from build123d import *

# Parameters (mm, degrees)
SKETCH_1_W          = 25
SKETCH_1_H          = 10
EXTRUDE_1_DEPTH     = 5
SKETCH_2_W          = 5
SKETCH_2_H          = 2
CUT_EXTRUDE_1_DEPTH = 10
SKETCH_4_R          = 1
CUT_EXTRUDE_2_DEPTH = 10


with BuildPart() as part:
    # 스케치1 → 보스-돌출1 (new body)
    with BuildSketch(Plane(origin=(0, 0, 0), x_dir=(0, 0, -1), z_dir=(1, 0, 0))):
        with Locations((12.5, 5)):
            Rectangle(SKETCH_1_W, SKETCH_1_H)
    extrude(amount=EXTRUDE_1_DEPTH)

    # 스케치2 → 컷-돌출1 (cut)
    with BuildSketch(Plane.ZY):
        with Locations((-2.5, 1)):
            Rectangle(SKETCH_2_W, SKETCH_2_H)
        with Locations((-2.5, 9)):
            Rectangle(SKETCH_2_W, SKETCH_2_H)
        with Locations((-22.5, 9)):
            Rectangle(SKETCH_2_W, SKETCH_2_H)
        with Locations((-22.5, 1)):
            Rectangle(SKETCH_2_W, SKETCH_2_H)
    extrude(amount=-CUT_EXTRUDE_1_DEPTH, mode=Mode.SUBTRACT)

    # 스케치4 → 컷-돌출2 (cut)
    with BuildSketch(Plane.ZY):
        with Locations((-4.292893219, 8.707106781)):
            Circle(SKETCH_4_R)
        with Locations((-4.292893219, 1.292893219)):
            Circle(SKETCH_4_R)
        with Locations((-20.707106781, 1.292893219)):
            Circle(SKETCH_4_R)
        with Locations((-20.707106781, 8.707106781)):
            Circle(SKETCH_4_R)
    extrude(amount=-CUT_EXTRUDE_2_DEPTH, mode=Mode.SUBTRACT)


solid = part.part
Read the model definition and answer for the solid it produces. Units are mm, in the model's axes. A direction names the side the tool comes from. Give positions to 0.01 mm unless a question says otherwise; leave off trailing zeros. Write each loop counter-clockwise with the first axis right and the second up, starting at its lowest first coordinate (ties: lowest second). Pieces come first, ordered by that corner, then holes. Notation, with made-up numbers: M 48.5,-5.5 L 83.5,-5.5 A32 ccw 83.5,24.5 Z; hole C -26.75,-25.5 d11. An arc over 180 degrees is marked long. One line per item, written item: value. Start each with the question number.
(1) Find section C-C (y = 8.5). Determine the outline of the cut face in (x, z).
(2) A tool of negligible diameter and unlimited length cuts with its end or side. For faces 1 (the flat face through (2, 2, -2)), 2 (the flat face through (2, 8, -23)), 3 (the flat face through (2, 8, -2)), from which of +Z, -Z, +X, -X, +Y, -Y can it reach the whole face along a straight path? Write none if from no direction.
(3) Find section B-B (z = -20.25). Determine the outline of the cut face in (x, y).
(4) Determine the mould class of faces 4 (the flat face through (2, 2, -23)), 5 (the flat face through (2, 5, -25)), 6 (the cylindrical face through (2, 2, -20)) for opening direction Z: pulls with the +Z half, pulls with the -Z half, needs draft (parallel to the pull), parting line crosses it, or undercut.
(5) Find the intervals of material crossed by line 1 (Y direction, x = 0.6, z = -21.5); line 2 (Z direction, x = 0.85, y = 9.5); line 3 (Z direction, x = 4.55, y = 1.25), in increasing order.
(6) Flat-ended cylindrical pins translate along their axes: pin 1 Ø1.1 at (x, z) = (2, -22.5) entering from +Y; pin 2 Ø1.8 at (x, z) = (1.5, -2) entering from -Y; pin 3 Ø0.6 at (x, y) = (1.5, 9.5) entering from +Z. Find the tip coordinate at first contact, or state that the pin passes through.
(7) Find section A-A (x = 2.9). Determine the outline of the cut face in (y, z).
Results below:
1. outline: M 0,-19.73 L 5,-19.73 L 5,-5.27 L 0,-5.27 Z
2. face 1: +Z, +X, -X, -Y
2. face 2: -Z, +X, -X, +Y
2. face 3: +Z, +X, -X, +Y
3. outline: M 0,2.18 L 5,2.18 L 5,7.82 L 0,7.82 Z
4. face 4: needs draft
4. face 5: pulls with the -Z half
4. face 6: undercut
5. line 1: y = 2 to 8
5. line 2: z = -20 to -5
5. line 3: z = -19.71 to -5.29
6. pin 1: stops at y = 8
6. pin 2: stops at y = 2
6. pin 3: stops at z = -5
7. outline: M 0,-20 L 0.59,-20 A1 cw 2,-21.41 L 2,-25 L 8,-25 L 8,-21.41 A1 cw 9.41,-20 L 10,-20 L 10,-5 L 9.41,-5 A1 cw 8,-3.59 L 8,0 L 2,0 L 2,-3.59 A1 cw 0.59,-5 L 0,-5 Z
